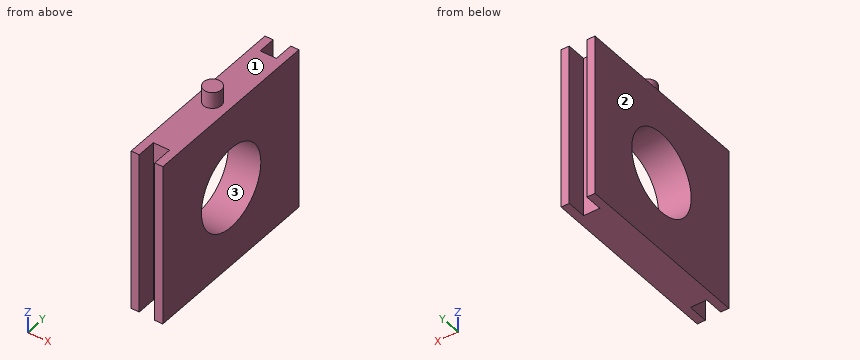
from build123d import *

# Parameters (mm, degrees)
F0_W     = 8.99
F0_H     = 10
F1_DEPTH = 1
F2_W     = 1.2572725254
F2_H     = 10
F2_W_2   = 1.20427544
F2_W_3   = 8.99
F3_DEPTH = 0.5
F4_W     = 1.095204528
F4_H     = 10
F4_W_2   = 8.99
F4_W_3   = 1.1806842821
F5_DEPTH = 0.5
F7_D     = 5
F8_R     = 0.546635634
F9_DEPTH = 1


with BuildPart() as f1:
    # F0 (on Right) → F1 (new body)
    with BuildSketch(Plane.YZ):
        with Locations((-15.5193753601, 5)):
            Rectangle(F0_W, F0_H)
    extrude(amount=F1_DEPTH)

    # F2 (on face) → F3 (join)
    with BuildSketch(Plane.YZ.offset(1)):
        with Locations((-20.6430116228, 5)):
            Rectangle(F2_W, F2_H)
        with Locations((-10.4222376401, 5)):
            Rectangle(F2_W_2, F2_H)
        with Locations((-15.5193753601, 5)):
            Rectangle(F2_W_3, F2_H)
    extrude(amount=F3_DEPTH)

    # F4 (on face) → F5 (join)
    with BuildSketch(Plane(origin=(0, 0, 0), x_dir=(0, -1, 0), z_dir=(-1, 0, 0))):
        with Locations((10.4767730961, 5)):
            Rectangle(F4_W, F4_H)
        with Locations((15.5193753601, 5)):
            Rectangle(F4_W_2, F4_H)
        with Locations((20.6047175011, 5)):
            Rectangle(F4_W_3, F4_H)
    extrude(amount=F5_DEPTH)

    # F7 (through all)
    with Locations(Plane(origin=(-0.5, 0, 0), x_dir=(0, -1, 0), z_dir=(-1, 0, 0))):
        with Locations((15.5227221549, 4.934320692)):
            Hole(F7_D / 2)

    # F8 (on face) → F9 (join)
    with BuildSketch(Plane.XY.offset(10)):
        with Locations((0.453364366, -15.6560353935)):
            Circle(F8_R)
    extrude(amount=F9_DEPTH)


solid = f1.part
CAD build for the part. Positions are in the model's coordinates, mm. Face numbers are marked on the shaded views. Coordinates: 2 decimals unless noted, no trailing zeros. Order: outer loops, then holes, each group sorted by start corner. A loop starts at its lowest first (then second) coordinate and runs counter-clockwise, first axis right, second up. Notation, with made-up numbers: (-4.75, 39) -> (52.25, 39) arc R14 ccw to (52.25, 55) -> close; hole circle Ø7 at (-27.5, 15). An arc over 180 degrees is marked (long way). Answer in a Markdown table with one row per item.
1) Band-saw the part on C-C (x = 0.2). List the corners of the cut face in (y, z).
Check values:
| item | result |
|---|---|
| outline | (-20.01, 0) -> (-11.02, 0) -> (-11.02, 10) -> (-15.17, 10) -> (-15.17, 11) -> (-16.14, 11) -> (-16.14, 10) -> (-20.01, 10) -> close; hole circle Ø5 at (-15.52, 4.93) |
2) Drill centre lines: line 1 (Y direction, x = -0.1, z = 5); line 2 (X direction, y = -20.5, z = 6.25); line 3 (Y direction, x = 0.5, z = 0.5). Where is each one in solid material? Low to high.
Check values:
| item | result |
|---|---|
| line 1 | -21.2 to -18.02, -13.02 to -9.93 |
| line 2 | -0.5 to 0, 1 to 1.5 |
| line 3 | -20.01 to -11.02 |
3) Band-saw the part on A-A (y = -10.25). List the corners of the cut face in (x, z), and give its area (3 significant figures).
Check values:
| item | result |
|---|---|
| outline | (-0.5, 0) -> (0, 0) -> (0, 10) -> (-0.5, 10) -> close; (1, 0) -> (1.5, 0) -> (1.5, 10) -> (1, 10) -> close |
| area | 10.0 mm2 |
4) Mould opens along Z. For the marked faces 1, 2 and 3 say: pulls with the +Z half, pulls with the -Z half, needs draft (parallel to the pull), parting line crosses it, or undercut.
Check values:
| item | result |
|---|---|
| face 1 | pulls with the +Z half |
| face 2 | needs draft |
| face 3 | undercut |
5) Flat gauge pins, fed straight in: P1, Ø0.8, axis at x = 0.5, z = 4, coming from the -Y side; P2, Ø1, axis at x = 1, y = -13, coming from the +Z side; P3, Ø0.6, axis at x = 0, z = 7.5, coming from the -Y side. Where does each tip first touch, or does it go through?
Check values:
| item | result |
|---|---|
| P1 | y = -20.01 |
| P2 | z = 10 |
| P3 | y = -21.2 |
6) Band-saw the part on D-D (z = 3.25). List the corners of the cut face in (x, y).
Check values:
| item | result |
|---|---|
| outline | (-0.5, -21.2) -> (0, -21.2) -> (0, -20.01) -> (1, -20.01) -> (1, -21.27) -> (1.5, -21.27) -> (1.5, -17.37) -> (-0.5, -17.37) -> close; (-0.5, -13.68) -> (1.5, -13.68) -> (1.5, -9.82) -> (1, -9.82) -> (1, -11.02) -> (0, -11.02) -> (0, -9.93) -> (-0.5, -9.93) -> close |
7) Band-saw the part on B-B (z = 9.5). List the corners of the cut face in (x, y), and give its area (3 significant figures).
Check values:
| item | result |
|---|---|
| outline | (-0.5, -21.2) -> (0, -21.2) -> (0, -20.01) -> (1, -20.01) -> (1, -21.27) -> (1.5, -21.27) -> (1.5, -9.82) -> (1, -9.82) -> (1, -11.02) -> (0, -11.02) -> (0, -9.93) -> (-0.5, -9.93) -> close |
| area | 20.3 mm2 |
